from build123d import *

# Parameters (mm, degrees)
SKETCH005_W  = 31
SKETCH005_H  = 11
PAD001_DEPTH = 0.5
SKETCH006_R  = 0.1


with BuildPart() as part:
    # Sketch005 → Pad001 (new body)
    with BuildSketch(Plane.XY):
        Rectangle(SKETCH005_W, SKETCH005_H)
    extrude(amount=PAD001_DEPTH)

    # AdditivePipe001: sweep along a path in Sketch008
    with BuildLine(Plane(origin=(-13.5, -3, 0), x_dir=(-1, 0, 0), z_dir=(0, 1, 0))) as additivepipe001_path:
        Line((0, 0), (2, 0))
        ThreePointArc((2, 0), (2.141421, 0.058579), (2.2, 0.2))
        Line((2.2, 0.2), (2.2, 2.7))
    # Sketch006 (on DatumPlane) → AdditivePipe001 (sweep)
    with BuildSketch(Plane(origin=(-13.5, 0, 0), x_dir=(0, -1, 0), z_dir=(-1, 0, 0))):
        with Locations((3, 0)):
            Circle(SKETCH006_R)
    additivepipe001 = sweep(path=additivepipe001_path.line)

    # Mirrored001: AdditivePipe001 across Sketch006 V_Axis
    add(additivepipe001.mirror(Plane(origin=(-13.5, 0, 0), x_dir=(-1, 0, 0), z_dir=(0, -1, 0))))


solid = part.part
Check sheet for the modelled part. Datum: model origin and axes. Units: mm. Give positions to 0.01 mm unless a question says otherwise; leave off trailing zeros. Write each loop counter-clockwise with the first axis right and the second up, starting at its lowest first coordinate (ties: lowest second). Pieces come first, ordered by that corner, then holes. Notation, with made-up numbers: (55, -5) -> (105, -5) arc R23 cw to (105, 4) -> close; hole circle Ø6 at (59, 59.25). An arc over 180 degrees is marked (long way). One line per item, written item: value. Start each with the question number.
Item 1: Material ranges on probe 1 along Z at (x, y) = (-5, -3), recorded low to high. Write a range as from..to.
Item 2: Section check C-C on x = -6. Record the cut outline in (y, z).
Item 3: Section check A-A on x = -14. Record the cut outline in (y, z), then the cut area to 3 significant figures.
Item 4: Section check B-B on y = -1. Record the cut outline in (x, z), then the cut area to 3 significant figures.
Item 5: Gauge pin test, flat ends, axial feed: pin 1 (1 mm diameter, centred on x = 7.5, y = -2, fed in from -Z); pin 2 (1.5 mm diameter, centred on y = -3.5, z = 1.5, fed in from +X); pin 3 (1 mm diameter, centred on x = -12, z = 2.5, fed in from -Y). Record the tip position at first contact, or that the pin passes through.
Results list:
1. probe 1: 0..0.5
2. outline: (-5.5, 0) -> (5.5, 0) -> (5.5, 0.5) -> (-5.5, 0.5) -> close
3. outline: (-5.5, 0) -> (-3.1, 0) arc R0.1 ccw to (-2.9, 0) -> (2.9, 0) arc R0.1 ccw to (3.1, 0) -> (5.5, 0) -> (5.5, 0.5) -> (-5.5, 0.5) -> close
3. area: 5.53 mm²
4. outline: (-15.5, 0) -> (15.5, 0) -> (15.5, 0.5) -> (-15.5, 0.5) -> close
4. area: 15.5 mm²
5. pin 1: z = 0
5. pin 2: x = -15.6
5. pin 3: through
